Part model, mm, in its own coordinate system. A direction names the side the tool comes from. Give positions to 0.01 mm unless a question says otherwise; leave off trailing zeros. Write each loop counter-clockwise with the first axis right and the second up, starting at its lowest first coordinate (ties: lowest second). Pieces come first, ordered by that corner, then holes.
from build123d import *

# Parameters (mm, degrees)
BOSS_EXTRU_1_DEPTH      = 60
BOSS_EXTRU_2_START      = 2.5
ESQUISSE3_W             = 15
ESQUISSE3_H             = 15
BOSS_EXTRU_2_DEPTH      = 50
ENL_V_START             = -10
ESQUISSE4_R             = 5.5
ENL_V_MAT_EXTRU_1_DEPTH = 105
ESQUISSE5_W             = 9.327942275
ESQUISSE5_H             = 15
BOSS_EXTRU_3_DEPTH      = 35
ESQUISSE12_W            = 95
ESQUISSE12_H            = 15
BOSS_EXTRU_9_DEPTH      = 5
ESQUISSE13_W            = 95
ESQUISSE13_H            = 15
BOSS_EXTRU_10_DEPTH     = 5
BOSS_EXTRU_12_DEPTH     = 20
ESQUISSE18_R            = 2.05
ENL_V_MAT_EXTRU_4_DEPTH = 50
ESQUISSE20_R            = 2
ENL_V_MAT_EXTRU_6_DEPTH = 32
BOSS_EXTRU_13_START     = 5
ESQUISSE21_R            = 2.5
BOSS_EXTRU_13_DEPTH     = 35


with BuildPart() as part:
    # Esquisse1 → Boss.-Extru.1 (new body)
    with BuildSketch(Plane.XY):
        Polygon((-29.816132576, -5), (20.183867424, -5), (20.183867424, 0), (-29.816132576, 0), (-79.816132576, -12.5), (-29.816132576, -25), (20.183867424, -25), (20.183867424, -20), (-29.816132576, -20), (-59.816132576, -12.5), align=None)
    extrude(amount=BOSS_EXTRU_1_DEPTH)

    # Esquisse3 → Boss.-Extru.2 (add)
    with BuildSketch(Plane.XY.offset(BOSS_EXTRU_2_START)):
        with Locations((-22.316132576, -12.5)):
            Rectangle(ESQUISSE3_W, ESQUISSE3_H)
    extrude(amount=BOSS_EXTRU_2_DEPTH)

    # Esquisse4 → Enlèv. mat.-Extru.1 (cut)
    with BuildSketch(Plane.XY.offset(ENL_V_START)):
        with Locations((-22.316132576, -12.5)):
            Circle(ESQUISSE4_R)
    extrude(amount=ENL_V_MAT_EXTRU_1_DEPTH, mode=Mode.SUBTRACT)

    # Esquisse5 → Boss.-Extru.3 (add)
    with BuildSketch(Plane.XY):
        with Locations((15.519896287, -12.5)):
            Rectangle(ESQUISSE5_W, ESQUISSE5_H)
    extrude(amount=BOSS_EXTRU_3_DEPTH)

    # Esquisse12 → Boss.-Extru.9 (add)
    with BuildSketch(Plane(origin=(0, 0, 0), x_dir=(1, 0, 0), z_dir=(0, 1, 0))):
        with Locations((17.683867424, -7.5)):
            Rectangle(ESQUISSE12_W, ESQUISSE12_H)
    extrude(amount=-BOSS_EXTRU_9_DEPTH)

    # Esquisse13 → Boss.-Extru.10 (add)
    with BuildSketch(Plane(origin=(0, -25, 0), x_dir=(-1, 0, 0), z_dir=(0, -1, 0))):
        with Locations((-17.683867424, -7.5)):
            Rectangle(ESQUISSE13_W, ESQUISSE13_H)
    extrude(amount=-BOSS_EXTRU_10_DEPTH)

    # Esquisse14 → Boss.-Extru.12 (add)
    with BuildSketch(Plane(origin=(65.183867424, 0, 0), x_dir=(0, 0, -1), z_dir=(1, 0, 0))):
        Polygon((0, 0), (-15, 0), (-15, -5), (0, -5), (10.113760869, 1), (50.113760869, 1), (50.113760869, 6), (10.113760869, 6), align=None)
        Polygon((-15, -25), (-15, -20), (0, -20), (10.113760869, -26), (50.113760869, -26), (50.113760869, -31), (10.113760869, -31), (0, -25), align=None)
    extrude(amount=-BOSS_EXTRU_12_DEPTH)

    # Esquisse18 → Enlèv. mat.-Extru.4 (cut)
    with BuildSketch(Plane(origin=(0, 6, 0), x_dir=(1, 0, 0), z_dir=(0, 1, 0))):
        with Locations(Location((60.269613545, 42.737284556, 0), (0, 0, 270))):  # turned: the seam where the file's is
            Circle(ESQUISSE18_R)
        with Locations(Location((60.269613545, 27.737284556, 0), (0, 0, 270))):  # turned: the seam where the file's is
            Circle(ESQUISSE18_R)
    extrude(amount=-ENL_V_MAT_EXTRU_4_DEPTH, mode=Mode.SUBTRACT)

    # Esquisse20 → Enlèv. mat.-Extru.6 (cut, through all)
    with BuildSketch(Plane(origin=(0, -25, 0), x_dir=(-1, 0, 0), z_dir=(0, -1, 0))):
        with Locations(Location((-15.612089386, -13.621364953, 0), (0, 0, 90))):  # turned: the seam where the file's is
            Circle(ESQUISSE20_R)
    extrude(amount=-ENL_V_MAT_EXTRU_6_DEPTH, mode=Mode.SUBTRACT)

    # Esquisse21 → Boss.-Extru.13 (add)
    with BuildSketch(Plane(origin=(0, -25, 0), x_dir=(-1, 0, 0), z_dir=(0, -1, 0)).offset(BOSS_EXTRU_13_START)):
        with Locations(Location((-15.612089386, -26.534383987, 0), (0, 0, 90))):  # turned: the seam where the file's is
            Circle(ESQUISSE21_R)
    extrude(amount=-BOSS_EXTRU_13_DEPTH)


solid = part.part
1) Saw through at A-A (x = 36). Write the cut outline in (y, z), and give its area (3 significant figures).
Check result:
outline: (-25, 0) - (-20, 0) - (-20, 15) - (-25, 15) - close; (-5, 0) - (0, 0) - (0, 15) - (-5, 15) - close
area: 150 mm2
2) Mould opens along Z. For faces 1 (the cylindrical face through (58.27, -28.47, -28.18)), 2 (the cylindrical face through (14.4, -12.68, 15.21)), 3 (the flat face through (-45.026, -8.802, 29.58)), 4 (the cylindrical face through (15.722, -27.535, 29.032)) say: +Z half, -Z half, draft (parallel to the pull), parting line (faces both ways), or undercut.
Check result:
face 1: undercut
face 2: undercut
face 3: draft
face 4: parting line
3) Saw through at D-D (z = 32.5). Write the cut outline in (x, y).
Check result:
outline: (-79.82, -12.5) - (-29.82, -25) - (20.18, -25) - (20.18, 0) - (-29.82, 0) - close; hole (-59.82, -12.5) - (-29.82, -20) - (-29.82, -5) - close; hole circle Ø11 at (-22.32, -12.5); hole (-14.82, -20) - (10.86, -20) - (10.86, -5) - (-14.82, -5) - close
4) Saw through at B-B (y = -15.5). Write the cut outline in (x, z), and give its area (3 significant figures).
Check result:
outline: (-67.82, 0) - (-47.82, 0) - (-47.82, 60) - (-67.82, 60) - close; (-29.82, 2.5) - (-26.93, 2.5) - (-26.93, 52.5) - (-29.82, 52.5) - close; (-17.71, 2.5) - (-14.82, 2.5) - (-14.82, 52.5) - (-17.71, 52.5) - close; (10.86, 0) - (20.18, 0) - (20.18, 35) - (10.86, 35) - close; hole circle Ø4 at (15.61, 13.62)
area: 1,800 mm2
5) 3-axis set-ups, long thin cutter, end or side, ignore diameter. For faces 5 (the flat face through (-14.816, -13, 27)), 6 (the flat face through (43, -23, 15)), 7 (the flat face through (-19, -7, 52.5)), 8 (the flat face through (55, 1, -30)), 9 (the flat face through (42, -5, 7)): which of +Z, -Z, +X, -X, +Y, -Y reach the whole face in a straight line?
Check result:
face 5: +Z, -Z
face 6: +Z, +X, +Y, -Y
face 7: +Z, +X
face 8: -Z, +X, -X
face 9: +Z, -Z, +X
6) Flat gauge pins, fed straight in: P1, Ø2.5, axis at x = 15.61, z = 13.62, coming from the +Y side; P2, Ø12, axis at y = -17.5, z = 31, coming from the +X side; P3, Ø2.5, axis at x = 34, y = -2.5, coming from the +Z side; P4, Ø12, axis at x = 32, z = 5.5, coming from the +Y side. Where does each tip first touch, or does it go through?
Check result:
P1: passes through
P2: stops at x = 20.18
P3: stops at z = 15
P4: stops at y = 0
7) Saw through at C-C (z = -19). Write the cut outline in (x, y).
Check result:
outline: (45.18, -31) - (65.18, -31) - (65.18, -26) - (45.18, -26) - close; (45.18, 1) - (65.18, 1) - (65.18, 6) - (45.18, 6) - close
8) Drill centre lines: L1, parallel to Y at x = 10, z = 9; L2, parallel to Y at x = 48, z = -30.5; L3, parallel to Z at x = -27, y = -22.5. Where is each one in solid material? Low to high.
Check result:
L1: y = -25 to -20, -5 to 0
L2: y = -31 to -26, 1 to 6
L3: z = 0 to 60
